from build123d import *

# Parameters (mm, degrees)
BOSS_EXTRUDE1_DEPTH           = 127
TAP_DRILL_FOR_8_32_TAP2_D     = 3.4544
TAP_DRILL_FOR_8_32_TAP2_DEPTH = 13.97
TAP_DRILL_FOR_8_32_TAP2_TIP   = 1.037806461
TAP_DRILL_FOR_8_32_TAP3_D     = 3.4544
TAP_DRILL_FOR_8_32_TAP3_DEPTH = 13.97
TAP_DRILL_FOR_8_32_TAP3_TIP   = 1.037806461


with BuildPart() as part:
    # Sketch1 → Boss-Extrude1 (new body)
    with BuildSketch(Plane(origin=(0, 0, 0), x_dir=(1, 0, 0), z_dir=(0, 1, 0))):
        Polygon((18.415, 0), (25.4, 0), (25.4, -12.7), (0, -12.7), (0, 0), (6.985, 0), (6.985, -7.065187713), (18.415, -7.065187713), align=None)
    extrude(amount=BOSS_EXTRUDE1_DEPTH)

    # Tap Drill for #8-32 Tap2
    with Locations(Plane(origin=(3.4925, 0, 6.35), x_dir=(0, 0, -1), z_dir=(0, -1, 0))):
        with Locations((0, 0), (0, 18.415)):
            Hole(TAP_DRILL_FOR_8_32_TAP2_D / 2, depth=TAP_DRILL_FOR_8_32_TAP2_DEPTH)
            with Locations((0, 0, -(TAP_DRILL_FOR_8_32_TAP2_DEPTH + TAP_DRILL_FOR_8_32_TAP2_TIP / 2))):  # 118° drill point
                Cone(0, TAP_DRILL_FOR_8_32_TAP2_D / 2, TAP_DRILL_FOR_8_32_TAP2_TIP, mode=Mode.SUBTRACT)

    # Tap Drill for #8-32 Tap3
    with Locations(Plane(origin=(3.4925, 127, 6.35), x_dir=(0, 0, 1), z_dir=(0, 1, 0))):
        with Locations((0, 0), (0, 18.415)):
            Hole(TAP_DRILL_FOR_8_32_TAP3_D / 2, depth=TAP_DRILL_FOR_8_32_TAP3_DEPTH)
            with Locations((0, 0, -(TAP_DRILL_FOR_8_32_TAP3_DEPTH + TAP_DRILL_FOR_8_32_TAP3_TIP / 2))):  # 118° drill point
                Cone(0, TAP_DRILL_FOR_8_32_TAP3_D / 2, TAP_DRILL_FOR_8_32_TAP3_TIP, mode=Mode.SUBTRACT)


solid = part.part
Check sheet for the modelled part. Datum: model origin and axes. Units: mm. A direction names the side the tool comes from. Round coordinates to 2 decimals unless told otherwise and drop trailing zeros. Loops run counter-clockwise (first coordinate to the right, second up) from the corner with the lowest first, then second, coordinate; pieces in that order, holes last. Notation, with made-up numbers: (-5, 33.5) -> (45, 33.5) arc R26 ccw to (45, 64.5) -> close; hole circle Ø9 at (-26, 20). An arc over 180 degrees is marked (long way). Put each result on its own line as item: value. Start each with the question number.
1. Section check A-A (z = 1.5). Enter the section's corners in (x, y) (3 decimals), plus the area to 3 significant figures.
2. Access from +Z, -Z, +X, -X, +Y, -Y to the whole of each face (thin tool, end or side, straight path). Record for faces 1 (the face through (20.22, 7.08, 5.98)), 2 (the face through (18.415, 63, 4)), 3 (the face through (25.4, 63, 6)), 4 (the face through (4, 119.9, 4.7)), 5 (the face through (3, 63, 0)).
3. Section check B-B (y = 74). Enter the section's corners in (x, z) (3 decimals).
4. Gauge pin test, flat end, axial feed: pin 1 (3 mm diameter, centred on x = 3.49, z = 6.35, fed in from -Y) (3 decimals). Record the tip position at first contact, or that the pin passes through.
5. Section check C-C (x = 10). Enter the section's corners in (y, z), plus the area to 3 significant figures.
6. Draft check along Z on faces 6 (the face through (22.2, 112.17, 6.31)), 7 (the face through (13, 63, 12.7)), 8 (the face through (13, 63, 7.065)), 9 (the face through (6.985, 63, 3)). Enter one of: +Z half, -Z half, draft (parallel to the pull), parting line (faces both ways), or undercut.
7. Scan lines: probe 1 along X at (y, z) = (5.25, 6.35) (3 decimals); probe 2 along X at (y, z) = (28.5, 3) (3 decimals); probe 3 along Z at (x, y) = (9.5, 98.5). Record each from-to range of solid material in increasing order.
Findings:
1. outline: (0, 0) -> (6.985, 0) -> (6.985, 127) -> (0, 127) -> close; (18.415, 0) -> (25.4, 0) -> (25.4, 127) -> (18.415, 127) -> close
1. area: 1,770 mm^2
2. face 1: -Y
2. face 2: -Z, +Y, -Y
2. face 3: +Z, -Z, +X, +Y, -Y
2. face 4: +Y
2. face 5: -Z, +X, -X, +Y, -Y
3. outline: (0, 0) -> (6.985, 0) -> (6.985, 7.065) -> (18.415, 7.065) -> (18.415, 0) -> (25.4, 0) -> (25.4, 12.7) -> (0, 12.7) -> close
4. pin 1: stops at y = 14.105
5. outline: (0, 7.07) -> (127, 7.07) -> (127, 12.7) -> (0, 12.7) -> close
5. area: 716 mm^2
6. face 6: undercut
6. face 7: +Z half
6. face 8: -Z half
6. face 9: draft
7. probe 1: x = 0 to 1.765, 5.22 to 6.985, 18.415 to 20.18, 23.635 to 25.4
7. probe 2: x = 0 to 6.985, 18.415 to 25.4
7. probe 3: z = 7.07 to 12.7
